CAD build for the part. Positions are in the model's coordinates, mm. Give positions to 0.01 mm unless a question says otherwise; leave off trailing zeros. Order: outer loops, then holes, each group sorted by start corner. A loop starts at its lowest first (then second) coordinate and runs counter-clockwise, first axis right, second up.
Item 1: Band-saw the part on B-B on z = 3.25. Give the cut face in (x, y).
Item 2: Band-saw the part on A-A on y = -4. Give the cut face in (x, z).
Item 3: Two-plate mould, pull along X, no slides. Class faces 1 (the flat face through (-2, -19, 27)), 2 (the flat face through (27.5, 0, 13)), 3 (the flat face through (0, -7.15, 1)): released by +X, released by -X, zero draft, split by the parting line, or undercut.
Item 4: Band-saw the part on D-D on z = 24.25. Give the cut face in (x, y), plus the area to 3 significant figures.
Item 5: Band-saw the part on C-C on x = 3. Give the cut face in (y, z), plus the area to 3 significant figures.
Item 6: Flat gauge pins, fed straight in: P1, Ø4, axis at x = -19.5, y = 10, coming from the +Z side; P2, Ø11, axis at x = 11.5, y = -2.5, coming from the +Z side; P3, Ø1.2, axis at x = -24, y = 15, coming from the +Z side. Where does each tip first touch, or does it go through?
Item 7: Wall check: L1, parallel to Y at x = 19, z = 2.75; L2, parallel to X at y = 6.5, z = 13.5; L3, parallel to Y at x = -19.5, z = 25. Give the ranges that are in metal, low to high.
```python
from build123d import *

# Parameters (mm, degrees)
F1_W     = 51
F1_H     = 36
F1_W_2   = 30.3
F1_H_2   = 14.3
F2_DEPTH = 2
F3_R     = 2.5
F4_DEPTH = 5
F5_DEPTH = 14
F0_W     = 55
F0_H     = 40
F0_W_2   = 51
F0_H_2   = 36
F6_DEPTH = 27
F7_SIZE  = 0.5


with BuildPart() as f2:
    # F1 (on face) → F2 (new body)
    with BuildSketch(Plane.XY):
        Rectangle(F1_W, F1_H)
        Rectangle(F1_W_2, F1_H_2, mode=Mode.SUBTRACT)
    extrude(amount=F2_DEPTH)

    # F3 (on face) → F4 (join)
    with BuildSketch(Plane.XY.offset(2)):
        with Locations((-19.15, 9.85)):
            Circle(F3_R)
        with Locations((18.85, 9.85)):
            Circle(F3_R)
        with Locations((18.85, -10.15)):
            Circle(F3_R)
        with Locations((-19.15, -10.15)):
            Circle(F3_R)
    extrude(amount=F4_DEPTH)

    # F3 (on face) → F5 (join)
    with BuildSketch(Plane.XY.offset(2)):
        Polygon((-21.5, 18), (-25.5, 18), (-25.5, 14), align=None)
        Polygon((-25.5, -14), (-25.5, -18), (-21.5, -18), align=None)
        Polygon((21.5, -18), (25.5, -18), (25.5, -14), align=None)
        Polygon((25.5, 14), (25.5, 18), (21.5, 18), align=None)
    extrude(amount=F5_DEPTH)

    # F0 (on Top) → F6 (join)
    with BuildSketch(Plane.XY):
        Rectangle(F0_W, F0_H)
        Rectangle(F0_W_2, F0_H_2, mode=Mode.SUBTRACT)
    extrude(amount=F6_DEPTH)

    # F7
    f7_edges = [f2.edges().sort_by_distance(p)[0] for p in [
        (0, 7.15, 2),
        (15.15, 0, 2),
        (0, -7.15, 2),
        (-15.15, 0, 2),
    ]]
    chamfer(f7_edges, length=F7_SIZE)


solid = f2.part
```
The answers:
1. outline: (-27.5, -20) - (27.5, -20) - (27.5, 20) - (-27.5, 20) - close; circle Ø5 at (-19.15, -10.15); circle Ø5 at (-19.15, 9.85); circle Ø5 at (18.85, -10.15); circle Ø5 at (18.85, 9.85); hole (-25.5, -14) - (-21.5, -18) - (21.5, -18) - (25.5, -14) - (25.5, 14) - (21.5, 18) - (-21.5, 18) - (-25.5, 14) - close
2. outline: (-27.5, 0) - (-15.15, 0) - (-15.15, 1.5) - (-15.65, 2) - (-25.5, 2) - (-25.5, 27) - (-27.5, 27) - close; (15.15, 0) - (27.5, 0) - (27.5, 27) - (25.5, 27) - (25.5, 2) - (15.65, 2) - (15.15, 1.5) - close
3. face 1: zero draft
3. face 2: released by +X
3. face 3: undercut
4. outline: (-27.5, -20) - (27.5, -20) - (27.5, 20) - (-27.5, 20) - close; hole (-25.5, -18) - (25.5, -18) - (25.5, 18) - (-25.5, 18) - close
4. area: 364 mm2
5. outline: (-20, 0) - (-7.15, 0) - (-7.15, 1.5) - (-7.65, 2) - (-18, 2) - (-18, 27) - (-20, 27) - close; (7.15, 0) - (20, 0) - (20, 27) - (18, 27) - (18, 2) - (7.65, 2) - (7.15, 1.5) - close
5. area: 151 mm2
6. P1: stops at z = 7
6. P2: stops at z = 2
6. P3: stops at z = 16
7. L1: y = -20 to -18, -12.65 to -7.65, 7.35 to 12.35, 18 to 20
7. L2: x = -27.5 to -25.5, 25.5 to 27.5
7. L3: y = -20 to -18, 18 to 20
